Input: part model. Units: mm. Frame: model coordinates. Round coordinates to 2 decimals unless told otherwise and drop trailing zeros. Order: outer loops, then holes, each group sorted by start corner. A loop starts at its lowest first (then second) coordinate and runs counter-clockwise, first axis right, second up. Notation, with made-up numbers: M 88.25,73.25 L 113.25,73.25 A21 ccw 113.25,92.25 Z; hole C -6.75,-16.75 d1. An arc over 180 degrees is marked long. One line per question, with ' | ' between items.
```python
from build123d import *

# Parameters (mm, degrees)
F0_R     = 3.812453
F1_DEPTH = 5.08


with BuildPart() as f1:
    # F0 (on Top) → F1 (new body)
    with BuildSketch(Plane.XY):
        with BuildLine():
            ThreePointArc((1.905218, 41.257359), (4.212179, 43.126849), (5.08, 45.966557))
            ThreePointArc((5.08, 45.966557), (-2.839904, 50.178605), (-1.904782, 41.257183))
            ThreePointArc((-1.904782, 41.257183), (0.000236, 40.886557), (1.905218, 41.257359))
        make_face()
        with Locations((0, 45.966557)):
            Circle(F0_R, mode=Mode.SUBTRACT)
        with BuildLine():
            ThreePointArc((1.905218, 41.257359), (0.000236, 40.886557), (-1.904782, 41.257183))
            Line((-1.904782, 41.257183), (-1.904782, 40.316892))
            Line((-1.904782, 40.316892), (1.905218, 40.316892))
            Line((1.905218, 40.316892), (1.905218, 41.257359))
        make_face()
        Polygon((1.905218, 40.316892), (-1.904782, 40.316892), (-1.904782, -99.383108), (0, -99.383108), (1.905218, -99.383108), align=None)
        with BuildLine():
            Line((0, -99.383108), (-1.904782, -99.383108))
            Line((-1.904782, -99.383108), (-1.904782, -99.893425))
            ThreePointArc((-1.904782, -99.893425), (-0.985979, -99.512898), (0, -99.383108))
        make_face()
        with BuildLine():
            Line((1.905218, -99.893677), (1.905218, -99.383108))
            Line((1.905218, -99.383108), (0, -99.383108))
            ThreePointArc((0, -99.383108), (0.986222, -99.512963), (1.905218, -99.893677))
        make_face()
        with BuildLine():
            ThreePointArc((1.905218, -99.893677), (0.986222, -99.512963), (0, -99.383108))
            ThreePointArc((0, -99.383108), (-0.985979, -99.512898), (-1.904782, -99.893425))
            ThreePointArc((-1.904782, -99.893425), (-1.905109, -106.492602), (3.81, -103.193108))
            ThreePointArc((3.81, -103.193108), (3.29962, -101.288217), (1.905218, -99.893677))
        make_face()
    extrude(amount=F1_DEPTH)


solid = f1.part
```
Item 1: Section query C-C, the plane y = -38.5. Return loops of the section in (x, z).
Report:
outline: M -1.9,0 L 1.91,0 L 1.91,5.08 L -1.9,5.08 Z
Item 2: Section query A-A, the plane x = 0. Return loops of the section in (y, z).
Report:
outline: M -107,0 L 42.15,0 L 42.15,5.08 L -107,5.08 Z; M 49.78,0 L 51.05,0 L 51.05,5.08 L 49.78,5.08 Z
Item 3: Section query B-B, the plane z = 1.65. Return loops of the section in (x, y).
Report:
outline: M -1.9,-99.89 A3.81 ccw long 3.81,-103.19 A3.81 ccw 1.91,-99.89 L 1.91,41.26 A5.08 ccw 5.08,45.97 A5.08 ccw long -1.9,41.26 Z; hole C 0,45.97 d7.62
Item 4: First-contact query: pin 1 (1.5 mm diameter, centred on y = -42, z = 2.5, fed in from -X); pin 2 (1.5 mm diameter, centred on x = -4, z = 1, fed in from +Y). Flat tips, straight axial feed; report the tip coordinate or a pass-through.
Report:
pin 1: x = -1.9 | pin 2: y = 49.87
Item 5: Mould query, pull axis X, two halves, no side actions, for faces 1 (the flat face through (0, -28, 0)), 2 (the flat face through (1.905, -30, 3)), 3 (the flat face through (-1.905, -28, 3)), 4 (the cylindrical face through (-0.826, 42.245, 2.504)). Classes: +X half, -X half, draft (parallel to the pull), parting line (faces both ways), or undercut.
Report:
face 1: draft | face 2: +X half | face 3: -X half | face 4: undercut
Item 6: Line query: line 1 along Y through (x, z) = (0, 2.6); line 2 along Y through (x, z) = (-2, 0.75); line 3 along X through (y, z) = (0.5, 2.8). Output: solid intervals per line, ascending. Write a range as from..to.
Report:
line 1: -107..42.15, 49.78..51.05 | line 2: -106.44..-99.95, 41.3..42.72, 49.21..50.64 | line 3: -1.9..1.91
